CAD build for the part. Positions are in the model's coordinates, mm. Coordinates: 2 decimals unless noted, no trailing zeros. One line per question, with ' | ' between items. Start each with the question number.
1. Probe line 1 (X direction, y = -10, z = 2.5); line 2 (X direction, y = 5.5, z = -0.5); line 3 (Y direction, x = -33, z = 1.25) (3 decimals). List the from-to ranges inside material, lowest first.
2. Flat gauge pins, fed straight in: P1, Ø20.5, axis at x = 30.87, y = 0, coming from the -Z side; P2, Ø3, axis at y = -8.5, z = 0.5, coming from the +X side; P3, Ø1, axis at y = -9.5, z = -1.5, coming from the -X side. Where does each tip first touch, or does it go through?
3. Band-saw the part on A-A, the plane y = 0. Give the number of separate pieces and of enclosed holes in the cut face, then the cut area to 3 significant figures.
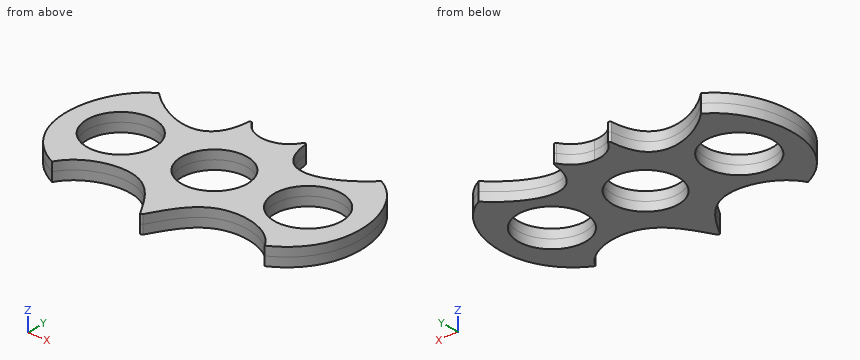
from build123d import *

# Parameters (mm, degrees)
F0_R     = 11.2811018545
F0_R_2   = 11
F1_DEPTH = 3
F2_R     = 0.5


with BuildPart() as f1:
    # F0 (on Top) → F1 (new body, symmetric)
    with BuildSketch(Plane.XY):
        with BuildLine():
            add(Edge.make_bspline(
                [(0, 20.6955336034), (4.176130984, 20.6701047719), (7.5252619572, 22.9629334062), (9.2714373022, 27.0963907242)],
                knots=[0, 0, 0, 0, 11.2663446392, 11.2663446392, 11.2663446392, 11.2663446392], degree=3))
            add(Edge.make_bspline(
                [(0, 20.6955336034), (-4.176130984, 20.6701047719), (-7.5252619572, 22.9629334062), (-9.2714373022, 27.0963907242)],
                knots=[0, 0, 0, 0, 11.2663446392, 11.2663446392, 11.2663446392, 11.2663446392], degree=3))
            add(Edge.make_bspline(
                [(-9.2714373022, 27.0963907242), (-10.252433829, 5.2865850739), (-29.1057825089, 14.5806018263), (-36.6129055619, 22.5558448583)],
                knots=[0, 0, 0, 0, 27.7159240033, 27.7159240033, 27.7159240033, 27.7159240033], degree=3))
            add(Edge.make_bspline(
                [(-36.6129055619, 22.5558448583), (-50.1396395266, 15.5486632138), (-55.6871630251, -12.4141490087), (-35.0454822183, -22.6485729218)],
                knots=[0, 0, 0, 0, 45.2315841285, 45.2315841285, 45.2315841285, 45.2315841285], degree=3))
            add(Edge.make_bspline(
                [(-35.0454822183, -22.6485729218), (-30.9359437749, -15.1486663001), (-9.8708452879, -9.8044342408), (-2.6448085105, -25.9140540409), (0, -30.179258436)],
                knots=[0, 0, 0, 0, 0.523784422, 1, 1, 1, 1], degree=3))
            add(Edge.make_bspline(
                [(35.0454822183, -22.6485729218), (30.9359437749, -15.1486663001), (9.8708452879, -9.8044342408), (2.6448085105, -25.9140540409), (0, -30.179258436)],
                knots=[0, 0, 0, 0, 0.523784422, 1, 1, 1, 1], degree=3))
            add(Edge.make_bspline(
                [(36.6129055619, 22.5558448583), (50.1396395266, 15.5486632138), (55.6871630251, -12.4141490087), (35.0454822183, -22.6485729218)],
                knots=[0, 0, 0, 0, 45.2315841285, 45.2315841285, 45.2315841285, 45.2315841285], degree=3))
            add(Edge.make_bspline(
                [(9.2714373022, 27.0963907242), (10.252433829, 5.2865850739), (29.1057825089, 14.5806018263), (36.6129055619, 22.5558448583)],
                knots=[0, 0, 0, 0, 27.7159240033, 27.7159240033, 27.7159240033, 27.7159240033], degree=3))
        make_face()
        with Locations((-30.8653861284, 0)):
            Circle(F0_R, mode=Mode.SUBTRACT)
        Circle(F0_R_2, mode=Mode.SUBTRACT)
        with Locations((30.8653861284, 0)):
            Circle(F0_R, mode=Mode.SUBTRACT)
    extrude(amount=F1_DEPTH, both=True)

    # F2
    f2_edges = [f1.edges().sort_by_distance(p)[0] for p in [
        (-9.271437, 27.096391, -1.5),
        (-9.271437, 27.096391, 1.5),
        (9.271437, 27.096391, -1.5),
        (9.271437, 27.096391, 1.5),
        (0, -30.179258, -1.5),
        (0, -30.179258, 1.5),
    ]]
    fillet(f2_edges, radius=F2_R)


solid = f1.part
Filled in:
1) line 1: x = -46.93 to -36.09, -25.64 to -4.58, 4.58 to 25.64, 36.09 to 46.93 | line 2: x = -48.09 to -40.71, -21.02 to -9.53, 9.53 to 21.02, 40.71 to 48.09 | line 3: y = -19.84 to -11.077, 11.077 to 19.315
2) P1: passes through | P2: stops at x = 47.89 | P3: stops at x = -47.29
3) separate pieces: 4 | enclosed holes: 0 | area: 181 mm²
